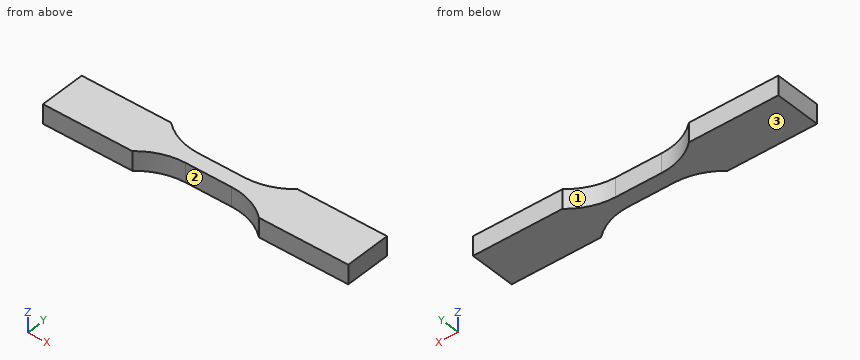
from build123d import *

# Parameters (mm, degrees)
BOSS_EXTRUDE1_DEPTH = 2
FILLET1_R           = 12.7
FILLET2_R           = 12.7


with BuildPart() as part:
    # Sketch1 → Boss-Extrude1 (new, symmetric)
    with BuildSketch(Plane.XY):
        Polygon((0, 0), (0, 9.53), (18.58, 9.53), (18.58, 6.355), (44.92, 6.355), (44.92, 9.53), (63.5, 9.53), (63.5, 0), (44.92, 0), (44.92, 3.175), (18.58, 3.175), (18.58, 0), align=None)
    extrude(amount=BOSS_EXTRUDE1_DEPTH, both=True)

    # Fillet1
    # the kernel refuses this fillet: 12.7 mm, written as the material it adds along each edge
    with BuildSketch(Plane(origin=(44.92, 3.175, 2), x_dir=(-1, 0, 0), z_dir=(0, 0, -1))) as fillet1_piece_1:
        with BuildLine():
            CenterArc((8.400260413, -12.7), FILLET1_R, 90, 41.409622109)
            Line((0, -3.175), (-0.168005208, -2.9845))
            ThreePointArc((-0.168005208, -2.9845), (-0.254, -1.5875), (-0.254, 0))
            Line((-0.254, 0), (0, 0.254))
            Line((0, 0.254), (8.400260413, 0.254))
            Line((8.400260413, 0.254), (8.400260413, 0))
        make_face()
    extrude(amount=4)
    with BuildSketch(Plane(origin=(18.58, 3.175, -2), x_dir=(0, -1, 0), z_dir=(0, 0, 1))) as fillet1_piece_2:
        with BuildLine():
            CenterArc((12.7, 8.400260413), FILLET1_R, 180, 41.409622109)
            Line((0, 8.400260413), (-0.254, 8.400260413))
            Line((-0.254, 8.400260413), (-0.254, 0))
            Line((-0.254, 0), (0, -0.254))
            ThreePointArc((0, -0.254), (1.5875, -0.254), (2.9845, -0.168005208))
            Line((2.9845, -0.168005208), (3.175, 0))
        make_face()
    extrude(amount=4)

    # Fillet2
    # the kernel refuses this fillet: 12.7 mm, written as the material it adds along each edge
    with BuildSketch(Plane(origin=(44.92, 6.355, 2), x_dir=(-1, 0, 0), z_dir=(0, 0, -1))) as fillet2_piece_1:
        with BuildLine():
            CenterArc((8.400260413, 12.7), FILLET2_R, 228.590377891, 41.409622109)
            Line((0, 3.175), (-0.168005208, 2.9845))
            ThreePointArc((-0.168005208, 2.9845), (-0.254, 1.5875), (-0.254, 0))
            Line((-0.254, 0), (0, -0.254))
            Line((0, -0.254), (8.400260413, -0.254))
            Line((8.400260413, -0.254), (8.400260413, 0))
        make_face()
    extrude(amount=4)
    with BuildSketch(Plane(origin=(18.58, 6.355, 2), x_dir=(0, 1, 0), z_dir=(0, 0, -1))) as fillet2_piece_2:
        with BuildLine():
            CenterArc((12.7, 8.400260413), FILLET2_R, 180, 41.409622109)
            Line((0, 8.400260413), (-0.254, 8.400260413))
            Line((-0.254, 8.400260413), (-0.254, 0))
            Line((-0.254, 0), (0, -0.254))
            ThreePointArc((0, -0.254), (1.5875, -0.254), (2.9845, -0.168005208))
            Line((2.9845, -0.168005208), (3.175, 0))
        make_face()
    extrude(amount=4)


solid = part.part
Source: CAD feature listing. Evaluate the final solid. Frame: model axes, mm. Face numbers are marked on the shaded views. A direction names the side the tool comes from. Round coordinates to 2 decimals unless told otherwise and drop trailing zeros. Order: outer loops, then holes, each group sorted by start corner. A loop starts at its lowest first (then second) coordinate and runs counter-clockwise, first axis right, second up. Notation, with made-up numbers: (12, -17) - (17, -17) arc R9 ccw to (17, -12) - close; hole circle Ø2 at (-2, 83). An arc over 180 degrees is marked (long way). Use a Markdown table: item, result. Add a question column.
1. Set-up query: the marked faces 1, 2 and 3. Return all of +Z, -Z, +X, -X, +Y, -Y with unobstructed straight access to the full face (end or side cutting, diameter ignored); none if empty.
2. Section query C-C (x = 28). Return the cut outline in (y, z) (3 decimals), then the cut area to 3 significant figures.
3. Line query: probe 1 along Y at (x, z) = (27, -1.45) (3 decimals); probe 2 along X at (y, z) = (0.5, -0.75); probe 3 along X at (y, z) = (1.5, 1.65). Output: solid intervals per line, ascending.
4. Section query A-A (y = 1.75). Return the cut outline in (x, z).
5. Section query D-D (x = 41.5). Return the cut outline in (y, z).
6. Section query B-B (z = 0.9). Return the cut outline in (x, y) (3 decimals).
7. First-contact query: pin 1 (2 mm diameter, centred on x = 29.5, z = 0, fed in from +Y) (3 decimals); pin 2 (4 mm diameter, centred on x = 31.5, y = 2.5, fed in from -Z). Flat tips, straight axial feed; report the tip coordinate or a pass-through.
Derived:
| question | item | result |
|---|---|---|
| 1 | face 1 | +Z, -Z, +Y |
| 1 | face 2 | +Z, -Z, -Y |
| 1 | face 3 | -Z, +X, -X, +Y, -Y |
| 2 | outline | (3.175, -2) - (6.355, -2) - (6.355, 2) - (3.175, 2) - close |
| 2 | area | 12.7 mm2 |
| 3 | probe 1 | 3.175 to 6.355 |
| 3 | probe 2 | 0 to 19.18, 44.32 to 63.5 |
| 3 | probe 3 | 0 to 20.68, 42.82 to 63.5 |
| 4 | outline | (0, -2) - (21.14, -2) - (21.14, 2) - (0, 2) - close; (42.36, -2) - (63.5, -2) - (63.5, 2) - (42.36, 2) - close |
| 5 | outline | (2.16, -2) - (7.37, -2) - (7.37, 2) - (2.16, 2) - close |
| 6 | outline | (0, 0) - (18.58, 0) arc R12.7 cw to (26.98, 3.175) - (36.52, 3.175) arc R12.7 cw to (44.92, 0) - (63.5, 0) - (63.5, 9.53) - (44.92, 9.53) arc R12.7 cw to (36.52, 6.355) - (26.98, 6.355) arc R12.7 cw to (18.58, 9.53) - (0, 9.53) - close |
| 7 | pin 1 | y = 6.355 |
| 7 | pin 2 | z = -2 |
